Verification items for the finished model (mm, model axes). A direction names the side the tool comes from. Give positions to 0.01 mm unless a question says otherwise; leave off trailing zeros. Write each loop counter-clockwise with the first axis right and the second up, starting at its lowest first coordinate (ties: lowest second). Pieces come first, ordered by that corner, then holes. Notation, with made-up numbers: (34.25, 89) - (66.25, 89) arc R33 ccw to (66.25, 127) - close; hole circle Ø2 at (-2.75, 70.25). An arc over 180 degrees is marked (long way). Answer as a JSON object with one key per item and string values. Group by question number.
Item 1: Go/stop test with flat-tipped pins: pin 1 (2 mm diameter, centred on x = 10, y = 1, fed in from +Z); pin 2 (1 mm diameter, centred on x = 4.5, y = 4, fed in from -Z); pin 3 (3 mm diameter, centred on y = 3.5, z = 41.5, fed in from +X). Record where each tip stops, or that it passes through.
Item 2: Sectioned sample at C-C, the plane x = 19.5. Record the boundary of the cut face in (y, z) (3 decimals), and give its area (3 significant figures).
Item 3: Tool access check on faces 1 (the face through (15, 3, -31.75)), 2 (the face through (4.83, 3.11, -52.22)), 3 (the face through (-5.4, 3.22, -56.24)), 4 (the face through (15, 3, 31.75)). Record the directions out of +Z, -Z, +X, -X, +Y, -Y that give a thin tool (end or side, any length) a straight path to the whole face; none if there is none.
Item 4: Sectioned sample at D-D, the plane z = -37. Record the boundary of the cut face in (x, y).
Item 5: Draft check along Y on faces 5 (the face through (6.35, 3, 43)), 6 (the face through (10.9, 3.3, -25.6)), 7 (the face through (6, 6.35, 1)). Enter one of: +Y half, -Y half, draft (parallel to the pull), parting line (faces both ways), or undercut.
Item 6: Scan lines: line 1 along Z through (x, y) = (0, 2); line 2 along Z through (x, y) = (22, 4.25); line 3 along Y through (x, z) = (16, -25). Record each from-to range of solid material in increasing order. Write a range as [from, to].
Item 7: Sectioned sample at B-B, the plane x = 0. Record the boundary of the cut face in (y, z).
Item 8: Sectioned sample at A-A, the plane z = 50.8. Record the boundary of the cut face in (x, y), and give its area (3 significant figures).
Autodesk Inventor part; units mm, degrees
ref_plane "Work Plane2" through (12.7, 0, 41.275) normal (1, 0, 0) x (0, 0, -1)
ref_plane "Work Plane3" through (14.2875, 0, 41.275) normal (1, 0, 0) x (0, 0, -1)
ref_plane "Work Plane1" through (12.7, 0, 41.275) normal (1, 0, 0) x (0, 0, -1)
sketch "Sketch1" plane through (0, 0, 0) normal (0, 1, 0) x (-1, 0, 0)
  line L0 (6.35, 57.15) -> (-6.35, 57.15)
  line L1 (-6.35, 57.15) -> (-6.35, -57.15)
  line L2 (-6.35, -57.15) -> (6.35, -57.15)
  line L3 (6.35, -57.15) -> (6.35, 57.15)
  circle A0 centre (0, 50.8) radius 3.556
  circle A1 centre (0, -50.8) radius 3.556
  point P0 (0, 0)
  dimension "d0" = 12.7
  dimension "d2" = 57.15
  dimension "d3" = 114.3
  dimension "d4" = 101.6
  dimension "d5" = 50.8
  dimension "d25" = 7.112
  dimension "d26" = 7.112
extrude "Extrusion1" add sketch "Sketch1" along normal blind 6.35
sketch "Sketch2" plane through (0, 0, 0) normal (0, -1, 0) x (1, 0, 0)
  circle A0 centre (0, -50.8) radius 3.556
  circle A1 centre (0, 50.8) radius 3.556
  point P0 (0, 0)
extrude "Extrusion2" [suppressed]
sketch "Sketch4" plane through (0, 6.35, 0) normal (0, 1, 0) x (1, 0, 0)
  circle A0 centre (-19.05, 15.1999) radius 3
  line L0 (-20.7085, 12.7) -> (-17.3915, 12.7)
  line L1 (-31.75, 12.7) -> (-6.35, 12.7)
  line L2 (-6.35, 57.15) -> (-6.35, -57.15)
  arc A1 (-16.521, 12.7) -> (-21.579, 12.7) centre (-19.05, 15.1999) ccw
  line L3 (-31.75, 12.7) -> (-6.35, 12.7)
  line L4 (-21.579, 12.7) -> (-20.7085, 12.7)
  line L5 (-17.3915, 12.7) -> (-16.521, 12.7)
  point P0 (0, 0)
  dimension "d18" = 6
  dimension "d19" = 3.317
  dimension "d20" = 0
  dimension "d21" = 12.7
  dimension "d22" = 7.112
extrude "Extrusion4" [suppressed]
mirror "Mirror1" [suppressed]
sketch "Sketch6" plane through (0, 0, 0) normal (0, -1, 0) x (1, 0, 0)
  line L0 (-6.35, 57.15) -> (6.35, 57.15)
  line L1 (6.35, 57.15) -> (12.7, 57.15)
  line L2 (12.7, 57.15) -> (12.7, -57.15)
  line L3 (12.7, -57.15) -> (6.35, -57.15)
  line L4 (6.35, -57.15) -> (6.35, 57.15)
  line L5 (6.35, -57.15) -> (-6.35, -57.15)
  point P0 (0, 0)
  dimension "d44" = 114.3
  dimension "d45" = 114.3
  dimension "d48" = 6.35
extrude "Extrusion6" [suppressed]
ref_plane "Work Plane2" through (12.7, 0, 41.275) normal (1, 0, 0) x (0, 0, -1)
ref_plane "Work Plane3" through (14.2875, 0, 41.275) normal (1, 0, 0) x (0, 0, -1)
ref_plane "Work Plane1" through (12.7, 0, 41.275) normal (1, 0, 0) x (0, 0, -1)
ref_plane "Work Plane4" through (12.7, 3.175, 41.275) normal (0, 1, 0) x (1, 0, 0)
sketch "Sketch11" plane through (0, 6.35, 0) normal (0, 1, 0) x (1, 0, 0)
  circle A0 centre (0, 50.8) radius 3.556
  line L0 (6.35, 57.15) -> (-6.35, 57.15)
  circle A1 centre (0, -48.895) radius 3.556
  point P0 (0, 0)
  dimension "d70" = 6.35
  dimension "d71" = 7.112
  dimension "d72" = 97.79
sketch "Sketch12" plane through (0, 0, 0) normal (0, -1, 0) x (1, 0, 0)
  circle A0 centre (0, 50.8) radius 3.556
  circle A1 centre (0, -50.8) radius 3.556
  circle A2 centre (0, -50.8) radius 1.651
  circle A3 centre (0, 50.8) radius 1.651
  point P0 (0, 0)
  dimension "d73" = 3.302
  dimension "d74" = 3.302
extrude "Extrusion11" [suppressed]
sketch "Sketch14" plane through (6.35, 0, 57.15) normal (1, 0, 0) x (0, 0, -1)
  circle A0 centre (6.35, 3.175) radius 1.4224
  line L0 (2.794, 6.35) -> (9.906, 6.35)
  line L1 (104.394, 6.35) -> (111.506, 6.35)
  line L2 (0, 0) -> (114.3, 0)
  point P0 (57.15, 0)
  point P1 (2.159, 1.27)
  point P2 (9.271, 1.27)
  point P3 (99.949, 1.27)
  point P4 (107.061, 1.27)
  dimension "d87" = 2.8448
  dimension "d99" = 3.175
  dimension "d100" = 6.35
  dimension "d101" = 7.112
  dimension "d102" = 3.556
extrude "Extrusion13" cut sketch "Sketch14" against normal up to next
thread "Thread3"
mirror "Mirror3" about plane through (0, 0, 0) normal (0, 0, 1) of "Extrusion13"
thread "Thread4"
fillet "Fillet1" radius 3.175 4 edges at (6.35, 3.175, 57.15) (-6.35, 3.175, 57.15) (6.35, 3.175, -57.15) (-6.35, 3.175, -57.15)
sketch "Sketch15" plane through (0, 6.35, 0) normal (0, 1, 0) x (1, 0, 0)
  line L0 (6.35, -53.975) -> (6.35, 53.975)
  line L1 (6.35, -31.75) -> (24.3434, -31.75)
  line L2 (24.3434, -31.75) -> (24.3434, 31.75)
  line L3 (24.3434, 31.75) -> (6.35, 31.75)
  line L4 (6.35, 31.75) -> (6.35, -31.75)
  point P0 (0, 0)
  dimension "d103" = 63.5
  dimension "d104" = 31.75
  dimension "d105" = 17.9934
extrude "Extrusion14" add sketch "Sketch15" against normal up to surface (6.35 mm away)
sketch "Sketch16" plane through (24.3434, 6.35, 31.75) normal (1, 0, 0) x (0, 0, -1)
  line L0 (0, 0) -> (0, -6.35)
  line L1 (0, 0) -> (63.5, 0)
  line L2 (0, -6.35) -> (63.5, -6.35)
  line L3 (31.75, -6.35) -> (31.75, 0)
  line L4 (85.725, 0) -> (-22.225, 0)
  point P0 (6.35, -3.175)
  point P1 (57.15, -3.175)
  dimension "d112" = 6.35
  dimension "d114" = 3.175
  dimension "d126" = 50.8
  dimension "d128" = 25.4
hole "Hole1" at (24.3434, 3.175, 25.4) at (24.3434, 3.175, -25.4) direction (-1, 0, 0) diameter 2.9464 depth 12.7 tip angle 118
thread "Thread5"
thread "Thread6"
equation "\"d26\" = d25"
equation "\"d45\" = d44"
equation "\"d74\" = d73"
equation "\"d99\" = 0.5 * d100"
equation "\"d102\" = 0.5 * d101"
properties part number "Slide rod connector" material "Aluminum 6061"
Geometry check:
{
 "1": {"pin 1": "z = 31.75", "pin 2": "z = -57.04", "pin 3": "x = 6.35"},
 "2": {"outline": "(0, -31.75) - (6.35, -31.75) - (6.35, 31.75) - (0, 31.75) - close; hole circle Ø2.946 at (3.175, -25.4); hole circle Ø2.946 at (3.175, 25.4)", "area": "390 mm^2"},
 "3": {"face 1": "-Z, +X, +Y, -Y", "face 2": "+X", "face 3": "-Z, -X, +Y, -Y", "face 4": "+Z, +X, +Y, -Y"},
 "4": {"outline": "(-6.35, 0) - (6.35, 0) - (6.35, 6.35) - (-6.35, 6.35) - close"},
 "5": {"face 5": "draft", "face 6": "undercut", "face 7": "+Y half"},
 "6": {"line 1": "[-57.15, -54.36], [-47.24, 47.24], [54.36, 57.15]", "line 2": "[-31.75, -26.41], [-24.39, 24.39], [26.41, 31.75]", "line 3": "[0, 1.76], [4.59, 6.35]"},
 "7": {"outline": "(0, -57.15) - (6.35, -57.15) - (6.35, -54.36) - (0, -54.36) - close; (0, -47.24) - (6.35, -47.24) - (6.35, 47.24) - (0, 47.24) - close; (0, 54.36) - (6.35, 54.36) - (6.35, 57.15) - (0, 57.15) - close"},
 "8": {"outline": "(-6.35, 0) - (-3.56, 0) - (-3.56, 6.35) - (-6.35, 6.35) - close; (3.56, 0) - (6.35, 0) - (6.35, 1.75) - (3.56, 1.75) - close; (3.56, 4.6) - (6.35, 4.6) - (6.35, 6.35) - (3.56, 6.35) - close", "area": "27.5 mm^2"}
}
